```python
from build123d import *

# Parameters (mm, degrees)
CROQUIS2_W              = 120
CROQUIS2_H              = 42
SALIENTE_EXTRUIR1_DEPTH = 10
REDONDEO1_R             = 6
CROQUIS3_W              = 65
CROQUIS3_H              = 95
SALIENTE_EXTRUIR2_DEPTH = 6
REDONDEO2_R             = 6
CROQUIS4_R              = 7.240565909
CORTAR_EXTRUIR1_DEPTH   = 11
CROQUIS6_R              = 35
CROQUIS6_R_2            = 30
EXTRUIR_L_MINA1_DEPTH   = 48
CROQUIS8_W              = 6
CROQUIS8_H              = 60.128808452
SALIENTE_EXTRUIR3_DEPTH = 36
CROQUIS9_R              = 6
SALIENTE_EXTRUIR4_DEPTH = 32.5
CROQUIS10_R             = 30
CORTAR_EXTRUIR3_DEPTH   = 49
CROQUIS11_W             = 3
CROQUIS11_H             = 67.611732644
CORTAR_EXTRUIR4_DEPTH   = 49


with BuildPart() as part:
    # Croquis2 → Saliente-Extruir1 (new body)
    with BuildSketch(Plane(origin=(0, 0, 0), x_dir=(1, 0, 0), z_dir=(0, 1, 0))):
        with Locations((0, -21)):
            Rectangle(CROQUIS2_W, CROQUIS2_H)
    extrude(amount=SALIENTE_EXTRUIR1_DEPTH)

    # Redondeo1
    redondeo1_edges = [part.edges().sort_by_distance(p)[0] for p in [
        (60, 5, 42),
        (-60, 5, 42),
        (-60, 5, 0),
        (60, 5, 0),
    ]]
    fillet(redondeo1_edges, radius=REDONDEO1_R)

    # Croquis3 → Saliente-Extruir2 (add)
    with BuildSketch(Plane.XY):
        with Locations((0, 57.5)):
            Rectangle(CROQUIS3_W, CROQUIS3_H)
    extrude(amount=SALIENTE_EXTRUIR2_DEPTH)

    # Redondeo2
    redondeo2_edges = [part.edges().sort_by_distance(p)[0] for p in [
        (32.5, 10, 3),
        (-32.5, 10, 3),
    ]]
    fillet(redondeo2_edges, radius=REDONDEO2_R)

    # Croquis4 → Cortar-Extruir1 (cut, through all)
    with BuildSketch(Plane(origin=(0, 10, 0), x_dir=(1, 0, 0), z_dir=(0, 1, 0))):
        with Locations((-38.5, -21)):
            Circle(CROQUIS4_R)
    cortar_extruir1 = extrude(amount=-CORTAR_EXTRUIR1_DEPTH, mode=Mode.SUBTRACT)

    # Simetría1: Cortar-Extruir1 across plane
    add(cortar_extruir1.mirror(Plane(origin=(0, 0, 0), x_dir=(0, 0, 1), z_dir=(1, 0, 0))), mode=Mode.SUBTRACT)

    # Croquis6 → Extruir-Lámina1 (add)
    with BuildSketch(Plane.XY.offset(-6)):
        with Locations((0, 105)):
            Circle(CROQUIS6_R)
        with Locations((0, 105)):
            Circle(CROQUIS6_R_2, mode=Mode.SUBTRACT)
    extrude(amount=EXTRUIR_L_MINA1_DEPTH)

    # Croquis8 → Saliente-Extruir3 (add)
    with BuildSketch(Plane.XY.offset(6)):
        with Locations((0, 40.064404226)):
            Rectangle(CROQUIS8_W, CROQUIS8_H)
    extrude(amount=SALIENTE_EXTRUIR3_DEPTH)

    # Croquis9 → Saliente-Extruir4 (add, symmetric)
    with BuildSketch(Plane(origin=(0, 0, 0), x_dir=(0, 0, -1), z_dir=(1, 0, 0))):
        with BuildLine():
            Line((0, 126.068220277), (0, 147))
            ThreePointArc((0, 147), (-14, 161), (-28, 147))
            Line((-28, 147), (-28, 119.03405794))
            Line((-28, 119.03405794), (0, 119.03405794))
            Line((0, 119.03405794), (0, 126.068220277))
        make_face()
        with Locations((-14, 147)):
            Circle(CROQUIS9_R, mode=Mode.SUBTRACT)
    extrude(amount=SALIENTE_EXTRUIR4_DEPTH, both=True)

    # Croquis10 → Cortar-Extruir3 (cut, through all)
    with BuildSketch(Plane.XY.offset(-6)):
        with Locations((0, 105)):
            Circle(CROQUIS10_R)
    extrude(amount=CORTAR_EXTRUIR3_DEPTH, mode=Mode.SUBTRACT)

    # Croquis11 → Cortar-Extruir4 (cut, through all)
    with BuildSketch(Plane.XY.offset(-6)):
        with Locations((0, 138.805866322)):
            Rectangle(CROQUIS11_W, CROQUIS11_H)
    extrude(amount=CORTAR_EXTRUIR4_DEPTH, mode=Mode.SUBTRACT)


solid = part.part
```
For this review, take the finished solid that the model builds, in its own axes (mm). A direction names the side the tool comes from. Give positions to 0.01 mm unless a question says otherwise; leave off trailing zeros. Order: outer loops, then holes, each group sorted by start corner. A loop starts at its lowest first (then second) coordinate and runs counter-clockwise, first axis right, second up.
1) Take a section at B-B (z = 11). Give the boundary of the cut face in (x, y).
2) The part is to be moulded in two halves that separate along Y. For faces 1 (the face through (-60, 5, 21)), 2 (the face through (-1, 0, 21)), 3 (the face through (17, 161, 14)), 4 (the face through (-32.5, 53, 3)), say which applies: released by +Y, released by -Y, zero draft, split by the parting line, or undercut.
3) For faces 5 (the face through (21, 139, 0)), 6 (the face through (-20, 139, 0)), 7 (the face through (21, 139, 28)), list the 3-axis set-ups (+Z, -Z, +X, -X, +Y, -Y) from which the entire face can be reached by the end or side of a thin tool; tool diameter is ignored.
4) Take a section at A-A (x = 24). Give the boundary of the cut face in (y, z).
5) Insertion check: pin 1 (22.5 mm diameter, centred on x = -14, y = 127, fed in from -Z); pin 2 (2 mm diameter, centred on y = 34, z = 27, fed in from +X); pin 3 (7 mm diameter, centred on y = 147, z = 14, fed in from +X); pin 4 (8 mm diameter, centred on y = 145, z = 10.5, fed in from +X). Each pin has a flat end and moves straight along its axis. Give the tip position at first contact, or say it passes through.
6) Take a section at C-C (y = 130). Give the boundary of the cut face in (x, z).
7) Take a section at D-D (y = 63). Give the boundary of the cut face in (x, z).
8) Wall thickness on line 1 (X direction, y = 7, z = 21); line 2 (X direction, y = 151.5, z = 5); line 3 (X direction, y = 105, z = 25): over which ranges is each line inside the solid? List them lowest first.
Derived:
1. outline: (-60, 0) - (60, 0) - (60, 10) - (3, 10) - (3, 70.13) arc R35 ccw to (32.06, 119.03) - (32.5, 119.03) - (32.5, 141.8) - (1.5, 141.8) - (1.5, 134.96) arc R30 cw (long way) to (-1.5, 134.96) - (-1.5, 141.8) - (-32.5, 141.8) - (-32.5, 119.03) - (-32.06, 119.03) arc R35 ccw to (-3, 70.13) - (-3, 10) - (-60, 10) - close; (-32.5, 152.2) - (-1.5, 152.2) - (-1.5, 160.67) - (-32.5, 160.67) - close; (1.5, 152.2) - (32.5, 152.2) - (32.5, 160.67) - (1.5, 160.67) - close
2. face 1: zero draft
2. face 2: released by -Y
2. face 3: released by +Y
2. face 4: undercut
3. face 5: -Z, +X, +Y
3. face 6: -Z, -X, +Y
3. face 7: +Z, +X, +Y
4. outline: (0, 0) - (79.52, 0) - (79.52, -6) - (87, -6) - (87, 42) - (79.52, 42) - (79.52, 6) - (10, 6) - (10, 42) - (0, 42) - close; (123, -6) - (130.48, -6) - (130.48, 0) - (147, 0) arc R14 ccw to (147, 28) - (130.48, 28) - (130.48, 42) - (123, 42) - close; hole circle Ø12 at (147, 14)
5. pin 1: stops at z = -6
5. pin 2: stops at x = 3
5. pin 3: passes through
5. pin 4: stops at x = 32.5
6. outline: (-32.5, 0) - (-24.49, 0) - (-24.49, -6) - (-16.58, -6) - (-16.58, 42) - (-24.49, 42) - (-24.49, 28) - (-32.5, 28) - close; (16.58, -6) - (24.49, -6) - (24.49, 0) - (32.5, 0) - (32.5, 28) - (24.49, 28) - (24.49, 42) - (16.58, 42) - close
7. outline: (-32.5, 0) - (32.5, 0) - (32.5, 6) - (3, 6) - (3, 42) - (-3, 42) - (-3, 6) - (-32.5, 6) - close
8. line 1: x = -60 to -45.74, -31.26 to 31.26, 45.74 to 60
8. line 2: x = -32.5 to -1.5, 1.5 to 32.5
8. line 3: x = -35 to -30, 30 to 35
